Geometry: final body of the model. Coordinates: model frame, mm. A direction names the side the tool comes from. Round coordinates to 2 decimals unless told otherwise and drop trailing zeros. Use one line per item in the form item = value. Start each with the question number.
1. Reachability of faces 4 (the face through (-1, 37, 2)), 5 (the face through (-1, -15, 3)), 6 (the face through (-28, -67, 0)) from +Z, -Z, +X, -X, +Y, -Y: full face, straight path, thin tool, end or side. Return the list, or none.
2. Draft query along Y for faces 1 (the face through (-9.764, -74.362, -1.232)), 2 (the face through (1, 37, 2)), 3 (the face through (0, 5, 1)). Return one class per face: pulls with the +Y half, pulls with the -Y half, needs draft (parallel to the pull), parting line crosses it, or undercut.
3. Pin query (flat end, axial travel): pin 1 Ø2 at (x, z) = (-32, 2) entering from -Y; pin 2 Ø1 at (y, z) = (-22, 1) entering from +X (3 decimals); pin 3 Ø0.8 at (x, z) = (1, 2.5) entering from -Y; pin 4 Ø4 at (x, y) = (0, -49.5) entering from +Z. Return the tip coordinate at first contact, or that it passes through.
4. Line query: L1, parallel to X at y = -0.5, z = -0.55; L2, parallel to Y at x = -12, z = 1.25. Output: solid intervals per line, ascending.
```python
from build123d import *

# Parameters (mm, degrees)
SKETCH_R           = 72
PAD_DEPTH          = 3
SKETCH001_R        = 75
PAD001_DEPTH       = 3
CHAMFER_SIZE       = 0.5
CHAMFER001_SIZE    = 0.5
POCKET_DEPTH       = 2
POLARPATTERN_COUNT = 3
POLARPATTERN_ANGLE = 180
SKETCH003_W        = 2
SKETCH003_H        = 72
POCKET001_DEPTH    = 2
SKETCH004_W        = 2
SKETCH004_H        = 5
POCKET002_DEPTH    = 4
FILLET_R           = 0.9


with BuildPart() as part:
    # Sketch → Pad (new body)
    with BuildSketch(Plane.XY):
        Circle(SKETCH_R)
    extrude(amount=PAD_DEPTH)

    # Sketch001 (on Face2 of Pad) → Pad001 (join)
    with BuildSketch(Plane(origin=(0, 0, 0), x_dir=(1, 0, 0), z_dir=(0, 0, -1))):
        Circle(SKETCH001_R)
    extrude(amount=PAD001_DEPTH)

    # Chamfer
    chamfer_edges = [part.edges().sort_by_distance(p)[0] for p in [
        (-75, 0, -3),
    ]]
    chamfer(chamfer_edges, length=CHAMFER_SIZE)

    # Chamfer001
    chamfer001_edges = [part.edges().sort_by_distance(p)[0] for p in [
        (-72, 0, 3),
    ]]
    chamfer(chamfer001_edges, length=CHAMFER001_SIZE)

    # Sketch002 (on Face4 of Chamfer001) → Pocket (cut)
    with BuildSketch(Plane.XY.offset(3)):
        Polygon((-60, -1.5), (-60, 1.5), (-55, 1.5), (-55, 0.5), (0, 0.5), (0, -0.5), (-55, -0.5), (-55, -1.5), align=None)
    pocket = extrude(amount=-POCKET_DEPTH, mode=Mode.SUBTRACT)

    # PolarPattern: Pocket ×3 about axis
    polarpattern_axis = Axis((0, 0, 3), (0, 0, 1))
    for i in range(1, POLARPATTERN_COUNT):
        add(pocket.rotate(polarpattern_axis, i * POLARPATTERN_ANGLE / (POLARPATTERN_COUNT - 1)), mode=Mode.SUBTRACT)

    # Sketch003 (on Face4 of PolarPattern) → Pocket001 (cut)
    with BuildSketch(Plane.XY.offset(3)):
        with Locations((0, 36)):
            Rectangle(SKETCH003_W, SKETCH003_H)
    extrude(amount=-POCKET001_DEPTH, mode=Mode.SUBTRACT)

    # Sketch004 (on Face8 of Pocket001) → Pocket002 (cut)
    with BuildSketch(Plane.XY.offset(3)):
        with Locations((0, 72.5)):
            Rectangle(SKETCH004_W, SKETCH004_H)
    extrude(amount=-POCKET002_DEPTH, mode=Mode.SUBTRACT)

    # Fillet
    fillet_edges = [part.edges().sort_by_distance(p)[0] for p in [
        (0, 70, 1),
        (0, 70, -1),
    ]]
    fillet(fillet_edges, radius=FILLET_R)


solid = part.part
```
Outcome:
q1.face_4 = +Z, +Y
q1.face_5 = +Z, +X, -X, +Y, -Y
q1.face_6 = +Z
q2.face_1 = parting line crosses it
q2.face_2 = needs draft
q2.face_3 = undercut
q3.pin_1 = -64.98
q3.pin_2 = 68.715
q3.pin_3 = -72
q3.pin_4 = 3
q4.L1 = -75 to 75
q4.L2 = -70.99 to -0.5, 0.5 to 70.99
